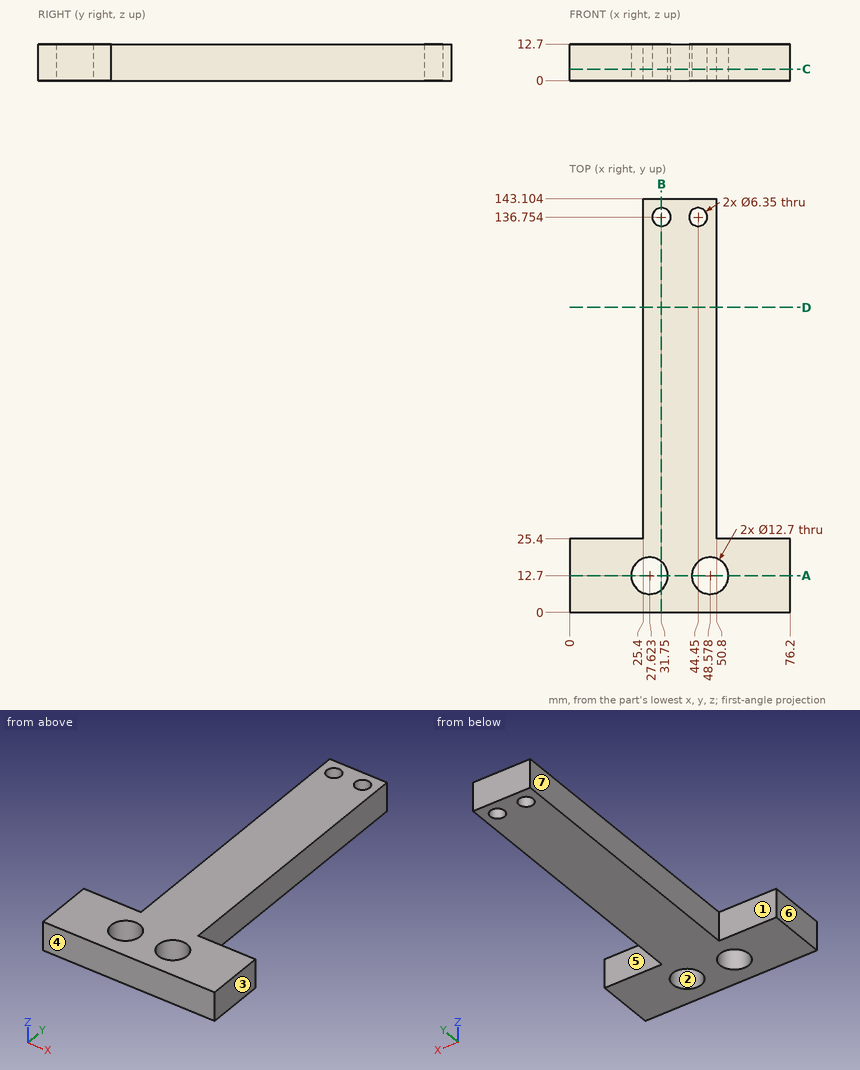
Job drawing, mm, ordinate dimensions from the low corner. One solid piece. A direction names the side the tool comes from. Coordinates: 2 decimals unless noted, no trailing zeros. Order: outer loops, then holes, each group sorted by start corner. A loop starts at its lowest first (then second) coordinate and runs counter-clockwise, first axis right, second up. Notation, with made-up numbers: (-39, 66.25) -> (-15, 66.25) arc R22 cw to (-15, 86.25) -> close; hole circle Ø8 at (72.5, 29.5). An arc over 180 degrees is marked (long way). Answer in a Markdown table with one row per item. Add a question column.
Q1. Band-saw the part on C-C, the plane z = 4. Give the number of separate pieces and of enclosed holes in the cut face, then the cut area to 3 significant figures.
Q2. Mould opens along Y. For the marked faces 1, 2, 3 and 4 say: +Y half, -Y half, draft (parallel to the pull), parting line (faces both ways), or undercut.
Q3. Wall check: line 1 along Y through (x, z) = (31.75, 6.5) (1 decimal); line 2 along X through (y, z) = (10, 3) (1 decimal); line 3 along Y through (x, z) = (27.5, 10.5). Give the ranges that are in metal, low to high. Write a range as [from, to].
Q4. Band-saw the part on B-B, the plane x = 31.75. List the corners of the cut face in (y, z) (1 decimal), then the cut area to 3 significant figures.
Q5. Band-saw the part on A-A, the plane y = 12.7. List the corners of the cut face in (x, z).
Q6. Which spindle directions (+Z, -Z, +X, -X, +Y, -Y) get a long thin tool onto all of the face, cutting with end or side? Do the marked faces 5, 6 and 7. Say none if no direction does.
Q7. Drop flat-ended pins along their axis: pin 1 (7.5 mm diameter, centred on x = 44.45, y = 136.75, fed in from -Z); pin 2 (4 mm diameter, centred on x = 17, z = 5.5, fed in from +Y); pin 3 (6 mm diameter, centred on y = 93.5, z = 1.5, fed in from -X); pin 4 (5.5 mm diameter, centred on x = 31.75, y = 136.75, fed in from +Z). Give the stop position or say it passes through.
Q8. Band-saw the part on D-D, the plane y = 105.5. List the corners of the cut face in (x, z), then the cut area to 3 significant figures.
Answers follow:
| question | item | result |
|---|---|---|
| 1 | separate pieces | 1 |
| 1 | enclosed holes | 4 |
| 1 | area | 4,610 mm^2 |
| 2 | face 1 | +Y half |
| 2 | face 2 | undercut |
| 2 | face 3 | draft |
| 2 | face 4 | -Y half |
| 3 | line 1 | [0, 7.9], [17.5, 133.6], [139.9, 143.1] |
| 3 | line 2 | [0, 21.9], [33.4, 42.8], [54.3, 76.2] |
| 3 | line 3 | [0, 6.35], [19.05, 143.1] |
| 4 | outline | (0, 0) -> (7.9, 0) -> (7.9, 12.7) -> (0, 12.7) -> close; (17.5, 0) -> (133.6, 0) -> (133.6, 12.7) -> (17.5, 12.7) -> close; (139.9, 0) -> (143.1, 0) -> (143.1, 12.7) -> (139.9, 12.7) -> close |
| 4 | area | 1,610 mm^2 |
| 5 | outline | (0, 0) -> (21.27, 0) -> (21.27, 12.7) -> (0, 12.7) -> close; (33.97, 0) -> (42.23, 0) -> (42.23, 12.7) -> (33.97, 12.7) -> close; (54.93, 0) -> (76.2, 0) -> (76.2, 12.7) -> (54.93, 12.7) -> close |
| 6 | face 5 | +Z, -Z, +X, +Y |
| 6 | face 6 | +Z, -Z, -X, +Y, -Y |
| 6 | face 7 | +Z, -Z, -X, +Y |
| 7 | pin 1 | z = 0 |
| 7 | pin 2 | y = 25.4 |
| 7 | pin 3 | x = 25.4 |
| 7 | pin 4 | through |
| 8 | outline | (25.4, 0) -> (50.8, 0) -> (50.8, 12.7) -> (25.4, 12.7) -> close |
| 8 | area | 323 mm^2 |
